Autodesk Inventor part; units mm, degrees
ref_plane "YZ Plane" through (0, 0, 0) normal (1, 0, 0) x (0, 1, 0)
ref_plane "XZ Plane" through (0, 0, 0) normal (0, 1, 0) x (-1, 0, 0)
ref_plane "XY Plane" through (0, 0, 0) normal (0, 0, 1) x (1, 0, 0)
sketch "草圖1" plane through (0, 0, 0) normal (0, 1, 0) x (-1, 0, 0)
  circle A0 centre (0, 0) radius 7.5
  circle A1 centre (0, 0) radius 9
  line L0 (7.5, 2.1585) -> (4.5, 2.1585)
  line L1 (4.5, 2.1585) -> (4.5, -2.1585)
  line L2 (4.5, -2.1585) -> (7.5, -2.1585)
  line L3 (7.5, -2.1585) -> (7.5, 2.1585)
  line L4 (7, 1) -> (4.5, 1)
  line L5 (4.5, 1) -> (4.5, -1)
  line L6 (4.5, -1) -> (7, -1)
  line L7 (7, -1) -> (7, 1)
  line L8 (0, 5.058) -> (0, -5.7034)
  line L9 (-7.5, 2.1585) -> (-4.5, 2.1585)
  line L10 (-4.5, 2.1585) -> (-4.5, -2.1585)
  line L11 (-4.5, -2.1585) -> (-7.5, -2.1585)
  line L12 (-7.5, -2.1585) -> (-7.5, 2.1585)
  line L13 (-7, 1) -> (-4.5, 1)
  line L14 (-4.5, -1) -> (-7, -1)
  line L15 (-7, -1) -> (-7, 1)
  point P0 (5.75, -1)
  point P1 (7.5, 0)
  point P2 (-7.1827, 2.1585)
  point P3 (7.1827, 2.1585)
  point P4 (4.5, 1)
  point P5 (7.1827, -2.1585)
  point P6 (-7.1827, -2.1585)
  point P7 (-4.5, 1)
  dimension "d0" = 15
  dimension "d1" = 18
  dimension "d2" = 2
  dimension "d3" = 1
  dimension "d4" = 0
  dimension "d5" = 2.5
  dimension "d28" = 3
extrude "擠出1" add sketch "草圖1" along normal blind 15 contours A0 L2 L1 L6 L7 L4 L0 | L3 L2 A0 | A0 L0 L3 | L9 L10 L13 L15 L14 L11 A0 | A0 L12 L9 | L11 L12 A0 | A1
sketch "草圖2" plane through (0, 15, 0) normal (0, 1, 0) x (1, 0, 0)
  circle A0 centre (0, 0) radius 15
  circle A1 centre (0, 0) radius 8
  dimension "d8" = 30
  dimension "d23" = 16
extrude "擠出2" add sketch "草圖2" along normal blind 2
sketch "草圖3" plane through (0, 0, 0) normal (0, -1, 0) x (1, 0, 0)
  circle A0 centre (0, 0) radius 11
  line L0 (-4.5, -2.1585) -> (-7.1827, -2.1585)
  circle A1 centre (0, 0) radius 7.5
extrude "擠出3" add sketch "草圖3" along normal blind 2
sketch "草圖4" plane through (0, -2, 0) normal (0, -1, 0) x (1, 0, 0)
  line L0 (-15, -15) -> (15, -15)
  line L1 (15, -15) -> (15, -5)
  line L2 (-15, -5) -> (-15, -15)
  circle A0 centre (0, 0) radius 7.5
  circle A1 centre (11, -10) radius 1.55
  circle A2 centre (-11, -10) radius 1.55
  line L3 (-15, -5) -> (15, -5)
  point P0 (0, -15)
  point P1 (-15, -10)
  point P2 (15, -10)
  dimension "d13" = 30
  dimension "d14" = 0
  dimension "d15" = 10
  dimension "d16" = 3.1
  dimension "d17" = 3.1
  dimension "d18" = 11
  dimension "d19" = 11
  dimension "d22" = 5
extrude "擠出4" add sketch "草圖4" along normal blind 2 contours L2 L3 A0 L1 L0 | L3 A0 picked at (1.4132, -5.3956)
sketch "草圖5" plane through (0, 0, 0) normal (0, -1, 0) x (1, 0, 0)
  line L0 (7, -1) -> (7, 1)
  line L1 (7, 1) -> (4.5, 1)
  line L2 (7, -1) -> (6.5, -1)
  line L3 (6.5, -1) -> (6.5, 1)
  line L4 (6.5, 1) -> (7, 1)
  line L5 (7, 1) -> (7, -1)
  line L6 (-7, -1) -> (-4.5, -1)
  line L7 (-7, 1) -> (-7, -1)
  line L8 (-6.5, -1) -> (-7, -1)
  line L9 (-7, -1) -> (-7, 1)
  line L10 (-7, 1) -> (-6.5, 1)
  line L11 (-6.5, 1) -> (-6.5, -1)
  point P0 (0, 0)
  dimension "d24" = 0.5
  dimension "d25" = 0.5
extrude "擠出5" add sketch "草圖5" against normal blind 15
properties part number "tmrEXCI"
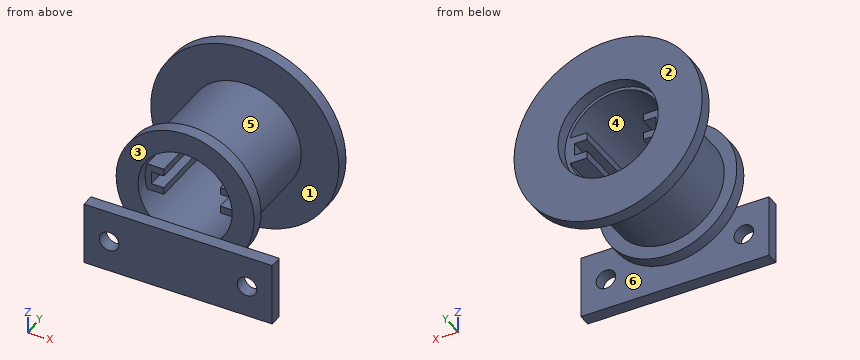
For this review, take the finished solid that the model builds, in its own axes (mm). Face numbers are marked on the shaded views. A direction names the side the tool comes from. Round coordinates to 2 decimals unless told otherwise and drop trailing zeros. Write each loop counter-clockwise with the first axis right and the second up, starting at its lowest first coordinate (ties: lowest second). Pieces come first, ordered by that corner, then holes. Notation, with made-up numbers: (61.5, 29) - (98.5, 29) arc R22 ccw to (98.5, 44) - close; hole circle Ø1 at (67.25, 23.25). An arc over 180 degrees is marked (long way). Write each question's results on one line, items separated by ' | '.
Item 1: For the marked faces 1, 2 and 3, list the 3-axis set-ups (+Z, -Z, +X, -X, +Y, -Y) from which the entire face can be reached by the end or side of a thin tool; tool diameter is ignored.
Calculated:
face 1: none | face 2: +Z, -Z, +X, -X, +Y | face 3: +Z, +X, -X, -Y
Item 2: Take a section at D-D on x = -10.5. State the section outline as (y, z) points.
Calculated:
outline: (-4, -15) - (-2, -15) - (-2, -11.47) - (-4, -11.47) - close; (-4, -8.53) - (-2, -8.53) - (-2, -5) - (-4, -5) - close; (-2, -3.28) - (0, -3.28) - (0, 3.28) - (-2, 3.28) - close; (15, -10.71) - (17, -10.71) - (17, 10.71) - (15, 10.71) - close
Item 3: To check wall thickness, follow line 1 along Y through (x, z) = (0.25, -11.25); line 2 along Y through (x, z) = (-8.75, -4.5); line 3 along Z through (x, y) = (-0.25, 16.25). State the ranges of each line that lie inside material, in increasing order. Write a range as from..to.
Calculated:
line 1: y = -4..-2, 15..17 | line 2: y = -2..0, 15..17 | line 3: z = -15..-8, 8..15
Item 4: Take a section at C-C on z = 0. State the section outline as (x, y) points.
Calculated:
outline: (-15, 15) - (-9, 15) - (-9, 0) - (-11, 0) - (-11, -2) - (-7.5, -2) - (-7.5, 0) - (-6.5, 0) - (-6.5, 15) - (-8, 15) - (-8, 17) - (-15, 17) - close; (6.5, 0) - (7.5, 0) - (7.5, -2) - (11, -2) - (11, 0) - (9, 0) - (9, 15) - (15, 15) - (15, 17) - (8, 17) - (8, 15) - (6.5, 15) - close
Item 5: For pin 1 (0.6 mm diameter, centred on x = 6, y = -3, fed in from +Z); pin 2 (2 mm diameter, centred on y = 14.5, z = 3.5, fed in from +X); pin 3 (17 mm diameter, centred on x = 0, z = 0, fed in from -Y); pin 4 (1.5 mm diameter, centred on x = -2.5, z = 5, fed in from -Y), all flat-tipped, find the tip position at first contact; note any pin that passes through.
Calculated:
pin 1: stops at z = -5 | pin 2: stops at x = 14.77 | pin 3: stops at y = -4 | pin 4: passes through
Item 6: Take a section at A-A on x = -2.5. State the section outline as (y, z) points.
Calculated:
outline: (-4, -15) - (-2, -15) - (-2, -10.71) - (0, -10.71) - (0, -8.65) - (15, -8.65) - (15, -14.79) - (17, -14.79) - (17, -7.6) - (15, -7.6) - (15, -7.07) - (-2, -7.07) - (-2, -5) - (-4, -5) - close; (-2, 7.07) - (15, 7.07) - (15, 7.6) - (17, 7.6) - (17, 14.79) - (15, 14.79) - (15, 8.65) - (0, 8.65) - (0, 10.71) - (-2, 10.71) - close
Item 7: Draft analysis for pull direction Z (two halves, no side actions). For the marked faces 4, 5 and 6, state which applies: pulls with the +Z half, pulls with the -Z half, needs draft (parallel to the pull), parting line crosses it, or undercut.
Calculated:
face 4: undercut | face 5: parting line crosses it | face 6: needs draft
Item 8: Take a section at B-B on y = 10.5. State the section outline as (x, z) points.
Calculated:
outline: circle Ø18 at (0, 0); hole (-7.18, -2.16) arc R7.5 ccw to (7.18, -2.16) - (4.5, -2.16) - (4.5, -1) - (6.5, -1) - (6.5, 1) - (4.5, 1) - (4.5, 2.16) - (7.18, 2.16) arc R7.5 ccw to (-7.18, 2.16) - (-4.5, 2.16) - (-4.5, 1) - (-6.5, 1) - (-6.5, -1) - (-4.5, -1) - (-4.5, -2.16) - close
